For this review, take the finished solid that the model builds, in its own axes (mm). A direction names the side the tool comes from. Give positions to 0.01 mm unless a question says otherwise; leave off trailing zeros. Loops run counter-clockwise (first coordinate to the right, second up) from the corner with the lowest first, then second, coordinate; pieces in that order, holes last.
```python
from build123d import *

# Parameters (mm, degrees)
F0_W        = 140
F0_H        = 40
F1_DEPTH    = 13.8
F2_R        = 7.9669047558
F3_T        = -2.5
F4_T1_DEPTH = 65


# Not quite as in the source:
# - a fillet or chamfer that OpenCascade refuses, or shapes differently, is made with other operations: its cross-section is extruded or revolved along the edge and cut away or added


with BuildPart() as f1:
    # F0 (on Front) → F1 (new body)
    with BuildSketch(Plane.XZ):
        with Locations((-0.0846795738, 4.6162967879)):
            Rectangle(F0_W, F0_H)
    extrude(amount=F1_DEPTH)

    # F2
    f2_edges = [f1.edges().sort_by_distance(p)[0] for p in [
        (69.91532, -6.9, 24.616297),
    ]]
    fillet(f2_edges, radius=F2_R)

    # F3
    f3_openings = [f1.faces().sort_by_distance(p)[0] for p in [
        (-0.25102, -13.8, 4.57187),
    ]]
    offset(amount=F3_T, openings=f3_openings)

    # F4: fillet of radius 5 on 1 edges, made by hand

    # F4_s2 → F4_t1 (cut)
    with BuildSketch(Plane.XY.offset(-27.8837032121)):
        with BuildLine():
            ThreePointArc((-70.0846795738, -8.8), (-68.6202134797, -12.3355339059), (-65.0846795738, -13.8))
            Line((-65.0846795738, -13.8), (-70.0846795738, -13.8))
            Line((-70.0846795738, -13.8), (-70.0846795738, -8.8))
        make_face()
    extrude(amount=F4_T1_DEPTH, mode=Mode.SUBTRACT)


solid = f1.part
```
Q1. Consider section D-D on y = -11.5. Give the boundary of the cut face in (x, z).
Answers:
outline: (-69.29, -15.38) - (69.92, -15.38) - (69.92, 16.65) arc R7.97 ccw to (61.95, 24.62) - (-69.29, 24.62) - close; hole (-67.58, -12.88) - (67.42, -12.88) - (67.42, 16.65) arc R5.47 ccw to (61.95, 22.12) - (-67.58, 22.12) - close
Q2. Consider section C-C on z = 4. Give the boundary of the cut face in (x, y), plus the area to 3 significant figures.
Answers:
outline: (-70.08, -8.8) arc R5 ccw to (-67.58, -13.13) - (-67.58, -2.5) - (67.42, -2.5) - (67.42, -13.8) - (69.92, -13.8) - (69.92, 0) - (-70.08, 0) - close
area: 402 mm2
Q3. Consider section B-B on x = -17.5. Give the boundary of the cut face in (y, z).
Answers:
outline: (-13.8, -15.38) - (0, -15.38) - (0, 24.62) - (-13.8, 24.62) - (-13.8, 22.12) - (-2.5, 22.12) - (-2.5, -12.88) - (-13.8, -12.88) - close
Q4. Machinability: for faces 1 (the cylindrical face through (67.643, -6.997, 22.221)), 2 (the flat face through (-1, -2.5, 5)), which of the approach directions +Z, -Z, +X, -X, +Y, -Y give a long, thin tool a straight path to every point of the face, cutting with its end or side? Answer none if there is none.
Answers:
face 1: +Z, +X, +Y, -Y
face 2: -Y
Q5. Consider section A-A on y = -3.75. Give the boundary of the cut face in (x, z).
Answers:
outline: (-70.08, -15.38) - (69.92, -15.38) - (69.92, 16.65) arc R7.97 ccw to (61.95, 24.62) - (-70.08, 24.62) - close; hole (-67.58, -12.88) - (67.42, -12.88) - (67.42, 16.65) arc R5.47 ccw to (61.95, 22.12) - (-67.58, 22.12) - close
Q6. Mouldability with a two-part tool opening along X and no side actions: class faces 3 (the flat face through (69.915, -7, 0)), 4 (the flat face through (-1, 0, 5)), 5 (the cylindrical face through (65.86, -8.23, 20.47)) as +X half, -X half, draft (parallel to the pull), parting line (faces both ways), or undercut.
Answers:
face 3: +X half
face 4: draft
face 5: undercut
Q7. For probe 1 along Z at (x, y) = (-16, -13); probe 2 along X at (y, z) = (-3.5, 14.5); probe 3 along Y at (x, z) = (21, -4), list the stretches that pass through material, from the lowest coordinate up.
Answers:
probe 1: z = -15.38 to -12.88, 22.12 to 24.62
probe 2: x = -70.08 to -67.58, 67.42 to 69.92
probe 3: y = -2.5 to 0
Q8. For pin 1 Ø8 at (x, z) = (-16, 0) entering from +Y; pin 2 Ø2 at (x, z) = (53.5, 1.5) entering from -Y, all flat-tipped, find the tip position at first contact; note any pin that passes through.
Answers:
pin 1: stops at y = 0
pin 2: stops at y = -2.5
